Geometry: final body of the model. Coordinates: model frame, mm. A direction names the side the tool comes from. Give positions to 0.01 mm unless a question says otherwise; leave off trailing zeros. Order: outer loops, then holes, each group sorted by start corner. A loop starts at its lowest first (then second) coordinate and runs counter-clockwise, first axis right, second up. Notation, with made-up numbers: M 3,-5 L 26,-5 A31 cw 26,21 Z; hole C 85.25,10.25 d8. An arc over 180 degrees is marked long. Use CSV: the item, a comma, the result in double quotes.
```python
from build123d import *

# Parameters (mm, degrees)
CUT_EXTRUDE1_DEPTH = 20
SKETCH3_R          = 1.475
CUT_EXTRUDE3_DEPTH = 8.9
CUT_EXTRUDE4_START = 2.8
SKETCH3_4_R        = 3
SKETCH3_4_R_2      = 1.475
CUT_EXTRUDE4_DEPTH = 6.1
CUT_EXTRUDE5_DEPTH = 2


with BuildPart() as part:
    # Sketch1 → Revolve1 (revolve)
    with BuildSketch(Plane(origin=(0, 0, 0), x_dir=(1, 0, 0), z_dir=(0, 1, 0))):
        Polygon((0, 0), (0, 11), (-7.2, 11), (-7.2, 9.2), (-59, 9.2), (-59, 0), align=None)
    revolve(axis=Axis((0, 0, 0), (-1, 0, 0)))

    # Sketch2 → Cut-Extrude1 (cut)
    with BuildSketch(Plane(origin=(0, 0, 0), x_dir=(0, 0, -1), z_dir=(1, 0, 0))):
        with BuildLine():
            ThreePointArc((2.527844932, 3.1), (0, 4), (-2.527844932, 3.1))
            Line((-2.527844932, 3.1), (2.527844932, 3.1))
        make_face()
        with BuildLine():
            Line((2.527844932, 3.1), (-2.527844932, 3.1))
            ThreePointArc((-2.527844932, 3.1), (-1.715899221, -3.613265817), (4, 0))
            ThreePointArc((4, 0), (3.613265817, 1.715899221), (2.527844932, 3.1))
        make_face()
    extrude(amount=-CUT_EXTRUDE1_DEPTH, mode=Mode.SUBTRACT)

    # Sketch3 → Cut-Extrude3 (cut, through all)
    with BuildSketch(Plane(origin=(0, 3.1, 0), x_dir=(-1, 0, 0), z_dir=(0, 1, 0))):
        with Locations((14, 0)):
            Circle(SKETCH3_R)
    extrude(amount=CUT_EXTRUDE3_DEPTH, mode=Mode.SUBTRACT)

    # Sketch3_4 → Cut-Extrude4 (cut, through all)
    with BuildSketch(Plane(origin=(0, 3.1, 0), x_dir=(-1, 0, 0), z_dir=(0, 1, 0)).offset(CUT_EXTRUDE4_START)):
        with Locations((14, 0)):
            Circle(SKETCH3_4_R)
        with Locations((14, 0)):
            Circle(SKETCH3_4_R_2, mode=Mode.SUBTRACT)
    extrude(amount=CUT_EXTRUDE4_DEPTH, mode=Mode.SUBTRACT)

    # Sketch2_6 → Cut-Extrude5 (cut)
    with BuildSketch(Plane(origin=(0, 0, 0), x_dir=(0, 0, -1), z_dir=(1, 0, 0))):
        with BuildLine():
            Line((0.5, 9.488630488), (0.5, 10.988630488))
            ThreePointArc((0.5, 10.988630488), (0, 11), (-0.5, 10.988630488))
            Line((-0.5, 10.988630488), (-0.5, 9.488630488))
            Line((-0.5, 9.488630488), (0.5, 9.488630488))
        make_face()
        with BuildLine():
            ThreePointArc((-0.5, -10.988630488), (0, -11), (0.5, -10.988630488))
            Line((0.5, -10.988630488), (0.5, -9.488630488))
            Line((0.5, -9.488630488), (-0.5, -9.488630488))
            Line((-0.5, -9.488630488), (-0.5, -10.988630488))
        make_face()
    extrude(amount=-CUT_EXTRUDE5_DEPTH, mode=Mode.SUBTRACT)


solid = part.part
```
1. Section A-A, the plane y = 8.5. Return the cut outline in (x, z), plus the area to 3 significant figures.
Answer:
outline,"M -59,-3.52 L -7.2,-3.52 L -7.2,-6.98 L 0,-6.98 L 0,6.98 L -7.2,6.98 L -7.2,3.52 L -59,3.52 Z; hole C -14,0 d6"
area,"437 mm2"
2. Section D-D, the plane x = -8. Return the cut outline in (y, z), plus the area to 3 significant figures.
Answer:
outline,"C 0,0 d18.4; hole C 0,0 d8"
area,"216 mm2"
3. Line query: line 1 (X direction, y = 7.65, z = 0); line 2 (Y direction, x = -6.5, z = 0); line 3 (X direction, y = 5.35, z = 0) (3 decimals). Output: solid intervals per line, ascending.
Answer:
line 1,"-59 to -17, -11 to 0"
line 2,"-11 to -4, 4 to 11"
line 3,"-59 to -15.475, -12.525 to 0"
4. Section C-C, the plane z = 7.5. Return the cut outline in (x, y), plus the area to 3 significant figures.
Answer:
outline,"M -59,-5.33 L -7.2,-5.33 L -7.2,-8.05 L 0,-8.05 L 0,8.05 L -7.2,8.05 L -7.2,5.33 L -59,5.33 Z"
area,"668 mm2"
5. Section B-B, the plane x = -14. Return the cut outline in (y, z) (3 decimals).
Answer:
outline,"M 3.718,-1.475 A4 cw long 3.718,1.475 L 5.9,1.475 L 5.9,3 L 8.697,3 A9.2 ccw long 8.697,-3 L 5.9,-3 L 5.9,-1.475 Z"
6. Pull-direction query (Y, two-part tool) for faces 1 (the face through (-1, -10, -0.5)), 2 (the face through (-15.3, 5.9, -1.3)), 3 (the face through (-20, 0, 0)); classes: +Y half, -Y half, draft (parallel to the pull), parting line (faces both ways), or undercut.
Answer:
face 1,"draft"
face 2,"+Y half"
face 3,"undercut"
7. Pin query (flat end, axial travel): pin 1 Ø1 at (x, z) = (-44.5, 0.5) entering from +Y; pin 2 Ø1.7 at (x, y) = (-1.5, -10.5) entering from -Z; pin 3 Ø0.5 at (x, y) = (-0.5, 10) entering from -Z. Return the tip coordinate at first contact, or that it passes through.
Answer:
pin 1,"y = 9.2"
pin 2,"z = -5.28"
pin 3,"z = -5.09"
8. Reachability of faces 4 (the face through (-15.407, 4.794, 0.443)), 5 (the face through (-1, 10, -0.5)), 6 (the face through (-1, -10, 0.5)) from +Z, -Z, +X, -X, +Y, -Y: full face, straight path, thin tool, end or side. Return the list, or none.
Answer:
face 4,"+Y"
face 5,"+X, +Y"
face 6,"+X, -Y"
